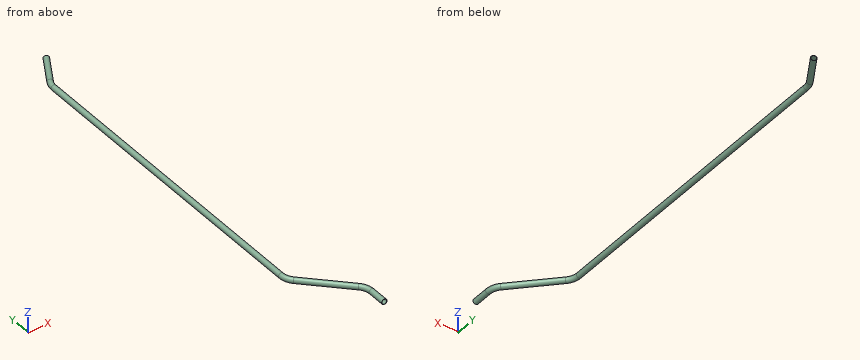
from build123d import *

# Parameters (mm, degrees)
SKETCH2_R   = 6.35
SKETCH2_R_2 = 5.5372


with BuildPart() as part:
    # Sweep1: sweep along a path in Sketch1
    with BuildLine(Plane.XY) as sweep1_path:
        Line((0, -253.63805), (0, -212.269586726))
        ThreePointArc((0, -212.269586726), (-2.900189811, -197.689347953), (-11.159231637, -185.328818363))
        Line((-11.159231637, -185.328818363), (-100.600768363, -95.887281637))
        ThreePointArc((-100.600768363, -95.887281637), (-108.859810189, -83.526752047), (-111.76, -68.946513274))
        Line((-111.76, -68.946513274), (-111.76, 682.844622495))
        ThreePointArc((-111.76, 682.844622495), (-110.461773982, 692.705628113), (-106.655567884, 701.894622495))
        Line((-106.655567884, 701.894622495), (-67.765909488, 769.253486726))
    # Sketch2 → Sweep1 (sweep)
    with BuildSketch(Plane(origin=(0, 0, 0), x_dir=(1, 0, 0), z_dir=(0, 1, 0))):
        with Locations((-111.76, 0)):
            Circle(SKETCH2_R)
        with Locations((-111.76, 0)):
            Circle(SKETCH2_R_2, mode=Mode.SUBTRACT)
    sweep(path=sweep1_path.line)


solid = part.part
Geometry: final body of the model. Coordinates: model frame, mm. Coordinates: 2 decimals unless noted, no trailing zeros. Loops run counter-clockwise (first coordinate to the right, second up) from the corner with the lowest first, then second, coordinate; pieces in that order, holes last. Notation, with made-up numbers: (52, 26) - (75, 26) arc R24 cw to (75, 64) - close; hole circle Ø9 at (69, -17.75). An arc over 180 degrees is marked (long way). One line per question, with ' | ' between items. Start each with the question number.
(1) Cut plane B-B on y = 287. Output: boundary loops of the cut face in (x, z), and give its area (3 significant figures).
(2) First-contact query: pin 1 (4 mm diameter, centred on y = 476, z = -4.5, fed in from +X); pin 2 (6 mm diameter, centred on y = -88.5, z = 1, fed in from -X); pin 3 (3 mm diameter, centred on x = -102.5, z = 1, fed in from +Y). Flat tips, straight axial feed; report the tip coordinate or a pass-through.
(3) Ray query, L1, parallel to Y at x = -85, z = -3.5; L2, parallel to Y at x = -78.5, z = 3.25; L3, parallel to X at y = -221, z = 0. Return the intervals inside material, ascending. Write a range as from..to.
Here are the results:
1) outline: circle Ø12.7 at (-111.76, 0); hole circle Ø11.07 at (-111.76, 0) | area: 30.4 mm²
2) pin 1: x = -105.92 | pin 2: x = -114.88 | pin 3: y = 724.27
3) L1: -118.98..-117.56, -105.42..-104, 728.81..730.82, 747.98..750 | L2: -125.7..-124.33, -111.65..-110.27, 739.75..741.7, 759.63..761.57 | L3: -6.35..-5.54, 5.54..6.35
